Can you work these out from the model? Positions are in its coordinate system, mm. A direction names the side the tool comes from. Give positions to 0.01 mm unless a question says otherwise; leave off trailing zeros. Order: outer loops, then holes, each group sorted by start corner. A loop starts at its lowest first (then second) coordinate and runs counter-clockwise, first axis right, second up.
```python
from build123d import *

# Parameters (mm, degrees)
ESQUISSE2_W         = 165
ESQUISSE2_H         = 165
BASE_DEPTH          = 30
ESQUISSE3_R         = 15
BLOC_MOTEUR_1_DEPTH = 80
ESQUISSE4_W         = 10
ESQUISSE4_H         = 22.360679774
ACCES_MOTEUR_DEPTH  = 37
ESQUISSE6_R         = 16.01
BLOC_MOTEUR_2_DEPTH = 37
ESQUISSE7_R         = 2.5
VIS_MOTEUR_DEPTH    = 121.467838032
ESQUISSE8_R         = 2.5
VIS_PATIN_DEPTH     = 121.467838032
ESQUISSE12_R        = 30
ESPACE_ROUE_DEPTH   = 10
ESQUISSE23_W        = 10
ESQUISSE23_H        = 30
VIDE_TIGE_DEPTH     = 10
VIDE_VIS_REACH      = 180.133
ESQUISSE25_R        = 2.5


with BuildPart() as part:
    # Esquisse2 → BASE (new body)
    with BuildSketch(Plane(origin=(0, 0, 0), x_dir=(1, 0, 0), z_dir=(0, 1, 0))):
        Rectangle(ESQUISSE2_W, ESQUISSE2_H)
    extrude(amount=BASE_DEPTH)

    # Esquisse3 → BLOC MOTEUR 1. (cut)
    with BuildSketch(Plane(origin=(82.5, 0, 0), x_dir=(0, 0, -1), z_dir=(1, 0, 0))):
        with Locations((50, 10)):
            Circle(ESQUISSE3_R)
    bloc_moteur_1 = extrude(amount=-BLOC_MOTEUR_1_DEPTH, mode=Mode.SUBTRACT)

    # Esquisse4 → ACCES MOTEUR (cut)
    with BuildSketch(Plane.XZ):
        with Locations((7.5, -50)):
            Rectangle(ESQUISSE4_W, ESQUISSE4_H)
    acces_moteur = extrude(amount=-ACCES_MOTEUR_DEPTH, mode=Mode.SUBTRACT)

    # Esquisse6 → BLOC MOTEUR 2 (cut)
    with BuildSketch(Plane(origin=(82.5, 0, 0), x_dir=(0, 0, -1), z_dir=(1, 0, 0))):
        with Locations((50, 10)):
            Circle(ESQUISSE6_R)
    bloc_moteur_2 = extrude(amount=-BLOC_MOTEUR_2_DEPTH, mode=Mode.SUBTRACT)

    # SYM BLOC MOTEUR: BLOC MOTEUR 1., ACCES MOTEUR, BLOC MOTEUR 2 across plane
    add(bloc_moteur_1.mirror(Plane(origin=(0, 0, 0), x_dir=(0, 0, 1), z_dir=(1, 0, 0))), mode=Mode.SUBTRACT)
    add(acces_moteur.mirror(Plane(origin=(0, 0, 0), x_dir=(0, 0, 1), z_dir=(1, 0, 0))), mode=Mode.SUBTRACT)
    add(bloc_moteur_2.mirror(Plane(origin=(0, 0, 0), x_dir=(0, 0, 1), z_dir=(1, 0, 0))), mode=Mode.SUBTRACT)

    # Esquisse7 → VIS MOTEUR (cut, through all)
    with BuildSketch(Plane.XZ):
        with Locations(Location((-64, -27.497196314, 0), (0, 0, 270))):
            Circle(ESQUISSE7_R)
        with Locations(Location((-24, -28.819660113, 0), (0, 0, 270))):
            Circle(ESQUISSE7_R)
        with Locations(Location((-24, -71.180339887, 0), (0, 0, 270))):
            Circle(ESQUISSE7_R)
        with Locations(Location((-64, -72.502803686, 0), (0, 0, 270))):
            Circle(ESQUISSE7_R)
    vis_moteur = extrude(amount=-VIS_MOTEUR_DEPTH, mode=Mode.SUBTRACT)

    # SYM VIS: VIS MOTEUR across plane
    add(vis_moteur.mirror(Plane(origin=(0, 0, 0), x_dir=(0, 0, 1), z_dir=(1, 0, 0))), mode=Mode.SUBTRACT)

    # Esquisse8 → VIS PATIN (cut, through all)
    with BuildSketch(Plane.XZ):
        with Locations(Location((-52.5, 52.5, 0), (0, 0, 270))):
            Circle(ESQUISSE8_R)
        with Locations(Location((52.5, 52.5, 0), (0, 0, 270))):
            Circle(ESQUISSE8_R)
    extrude(amount=-VIS_PATIN_DEPTH, mode=Mode.SUBTRACT)

    # Esquisse12 → ESPACE ROUE (cut)
    with BuildSketch(Plane.ZY.offset(82.5)):
        with Locations((-50, 10)):
            Circle(ESQUISSE12_R)
    espace_roue = extrude(amount=-ESPACE_ROUE_DEPTH, mode=Mode.SUBTRACT)

    # SYM ESPACE ROUE: ESPACE ROUE across plane
    add(espace_roue.mirror(Plane(origin=(0, 0, 0), x_dir=(0, 0, 1), z_dir=(1, 0, 0))), mode=Mode.SUBTRACT)

    # Esquisse23 → VIDE TIGE (cut)
    with BuildSketch(Plane(origin=(82.5, 0, 0), x_dir=(0, 0, -1), z_dir=(1, 0, 0))):
        with Locations((-72.5, 15)):
            Rectangle(ESQUISSE23_W, ESQUISSE23_H)
        with Locations((7.5, 15)):
            Rectangle(ESQUISSE23_W, ESQUISSE23_H)
    vide_tige = extrude(amount=-VIDE_TIGE_DEPTH, mode=Mode.SUBTRACT)

    # SYM TIGE: VIDE TIGE across plane
    add(vide_tige.mirror(Plane(origin=(0, 0, 0), x_dir=(0, 0, 1), z_dir=(1, 0, 0))), mode=Mode.SUBTRACT)

    # Esquisse25 → VIDE VIS (cut, up to next)
    with BuildSketch(Plane(origin=(72.5, 0, 0), x_dir=(0, 0, -1), z_dir=(1, 0, 0)), mode=Mode.PRIVATE) as vide_vis_sk1:
        with Locations((-72.5, 25)):
            Circle(ESQUISSE25_R)
    vide_vis_tool1 = extrude(vide_vis_sk1.sketch, amount=-VIDE_VIS_REACH, mode=Mode.PRIVATE) & part.part
    # Esquisse25 → VIDE VIS (cut, up to next)
    with BuildSketch(Plane(origin=(72.5, 0, 0), x_dir=(0, 0, -1), z_dir=(1, 0, 0)), mode=Mode.PRIVATE) as vide_vis_sk2:
        with Locations((-72.5, 15)):
            Circle(ESQUISSE25_R)
    vide_vis_tool2 = extrude(vide_vis_sk2.sketch, amount=-VIDE_VIS_REACH, mode=Mode.PRIVATE) & part.part
    # Esquisse25 → VIDE VIS (cut, up to next)
    with BuildSketch(Plane(origin=(72.5, 0, 0), x_dir=(0, 0, -1), z_dir=(1, 0, 0)), mode=Mode.PRIVATE) as vide_vis_sk3:
        with Locations((-72.5, 5)):
            Circle(ESQUISSE25_R)
    vide_vis_tool3 = extrude(vide_vis_sk3.sketch, amount=-VIDE_VIS_REACH, mode=Mode.PRIVATE) & part.part
    # Esquisse25 → VIDE VIS (cut, up to next)
    with BuildSketch(Plane(origin=(72.5, 0, 0), x_dir=(0, 0, -1), z_dir=(1, 0, 0)), mode=Mode.PRIVATE) as vide_vis_sk4:
        with Locations(Location((7.5, 5, 0), (0, 0, 180))):
            Circle(ESQUISSE25_R)
    vide_vis_tool4 = extrude(vide_vis_sk4.sketch, amount=-VIDE_VIS_REACH, mode=Mode.PRIVATE) & part.part
    # Esquisse25 → VIDE VIS (cut, up to next)
    with BuildSketch(Plane(origin=(72.5, 0, 0), x_dir=(0, 0, -1), z_dir=(1, 0, 0)), mode=Mode.PRIVATE) as vide_vis_sk5:
        with Locations(Location((7.5, 25, 0), (0, 0, 180))):
            Circle(ESQUISSE25_R)
    vide_vis_tool5 = extrude(vide_vis_sk5.sketch, amount=-VIDE_VIS_REACH, mode=Mode.PRIVATE) & part.part
    # Esquisse25 → VIDE VIS (cut, up to next)
    with BuildSketch(Plane(origin=(72.5, 0, 0), x_dir=(0, 0, -1), z_dir=(1, 0, 0)), mode=Mode.PRIVATE) as vide_vis_sk6:
        with Locations(Location((7.5, 15, 0), (0, 0, 180))):
            Circle(ESQUISSE25_R)
    vide_vis_tool6 = extrude(vide_vis_sk6.sketch, amount=-VIDE_VIS_REACH, mode=Mode.PRIVATE) & part.part
    add(vide_vis_tool1.solids().sort_by_distance((72.5, 25, 72.5))[0], mode=Mode.SUBTRACT)
    add(vide_vis_tool2.solids().sort_by_distance((72.5, 15, 72.5))[0], mode=Mode.SUBTRACT)
    add(vide_vis_tool3.solids().sort_by_distance((72.5, 5, 72.5))[0], mode=Mode.SUBTRACT)
    add(vide_vis_tool4.solids().sort_by_distance((72.5, 5, -7.5))[0], mode=Mode.SUBTRACT)
    add(vide_vis_tool5.solids().sort_by_distance((72.5, 25, -7.5))[0], mode=Mode.SUBTRACT)
    add(vide_vis_tool6.solids().sort_by_distance((72.5, 15, -7.5))[0], mode=Mode.SUBTRACT)


solid = part.part
```
1) If I drill on line 1 (Y direction, x = -6, z = -7.5); line 2 (X direction, y = 12, z = 52.5); line 3 (X direction, y = 4.5, z = -74), over which ranges is the centre line in solid material (lowest first)?
2) Suppose I cut it at A-A (z = -7.5). Please give me the cut outline in (x, y).
3) Suppose I cut it at D-D (x = -52.5). Please give me the cut outline in (y, z).
4) I'm going to push flat-ended pins straight in: pin 1 Ø5 at (y, z) = (9, -6) entering from +X; pin 2 Ø4 at (y, z) = (25, 72.5) entering from +X; pin 3 Ø9 at (y, z) = (9.5, -41.5) entering from -X; pin 4 Ø8 at (y, z) = (8, -51.5) entering from +X. Where does each tip first touch, or does it pass through?
5) We'd pull the mould along Y, two halves only. Please class faces 5 (the face through (77.57, 16.032, -79.387)), 6 (the face through (-23.89, 14.79, -68.683)), 7 (the face through (77.57, 15.591, -20.526)): +Y half, -Y half, draft (parallel to the pull), parting line (faces both ways), or undercut.
6) Suppose I cut it at B-B (x = 64). Give the number of separate pieces and of enclosed holes in the cut face, and give its area (3 significant figures).
7) Which directions (+Z, -Z, +X, -X, +Y, -Y) give clear straight access to the entire face, cutting with the end or side of a thin tool? Please do faces 1 (the face through (-24, 25, -50)), 2 (the face through (78, 15, -12.5)), 3 (the face through (-78, 15, -2.5)), 4 (the face through (7, 25, -38.82)).
8) Suppose I cut it at C-C (z = -50). Please give me the cut outline in (x, y).
Results:
1. line 1: y = 0 to 2.5, 7.5 to 12.5, 17.5 to 22.5, 27.5 to 30
1. line 2: x = -82.5 to -55, -50 to 50, 55 to 82.5
1. line 3: x = -72.5 to -66, -62 to 62, 66 to 72.5
2. outline: (-72.5, 0) - (72.5, 0) - (72.5, 2.5) - (-72.5, 2.5) - close; (-72.5, 7.5) - (72.5, 7.5) - (72.5, 12.5) - (-72.5, 12.5) - close; (-72.5, 17.5) - (72.5, 17.5) - (72.5, 22.5) - (-72.5, 22.5) - close; (-72.5, 27.5) - (72.5, 27.5) - (72.5, 30) - (-72.5, 30) - close
3. outline: (0, -82.5) - (30, -82.5) - (30, 50) - (0, 50) - (0, -37.5) arc R16.01 cw (long way) to (0, -62.5) - close; (0, 55) - (30, 55) - (30, 82.5) - (0, 82.5) - close; hole circle Ø5 at (5, -7.5); hole circle Ø5 at (5, 72.5); hole circle Ø5 at (15, -7.5); hole circle Ø5 at (15, 72.5); hole circle Ø5 at (25, -7.5); hole circle Ø5 at (25, 72.5)
4. pin 1: stops at x = 72.5
4. pin 2: passes through
4. pin 3: stops at x = -2.5
4. pin 4: stops at x = 2.5
5. face 5: undercut
5. face 6: draft
5. face 7: undercut
6. separate pieces: 3
6. enclosed holes: 6
6. area: 3,830 mm2
7. face 1: -X
7. face 2: +X, +Y, -Y
7. face 3: -X, +Y, -Y
7. face 4: +Y, -Y
8. outline: (-72.5, 26.01) - (-45.5, 26.01) - (-45.5, 25) - (-12.5, 25) - (-12.5, 30) - (-72.5, 30) - close; (-2.5, 0) - (2.5, 0) - (2.5, 30) - (-2.5, 30) - close; (12.5, 25) - (45.5, 25) - (45.5, 26.01) - (72.5, 26.01) - (72.5, 30) - (12.5, 30) - close
